Work out the finished part from the listing and answer in its coordinate system (mm). Coordinates: 2 decimals unless noted, no trailing zeros. Order: outer loops, then holes, each group sorted by start corner. A loop starts at its lowest first (then second) coordinate and runs counter-clockwise, first axis right, second up. Notation, with made-up numbers: (-14.75, 28.5) -> (-1.75, 28.5) arc R12 ccw to (-1.75, 33.5) -> close; hole circle Ø6 at (10, -36). An arc over 180 degrees is marked (long way). Answer as CSV lines item,"result". Start each with the question number.
Item 1: Straight lines are drawn through the part: L1, parallel to Z at x = -1.25, y = 1.2; L2, parallel to Y at x = 1, z = -8.25; L3, parallel to Y at x = -0.5, z = -12. For each, find the intervals that lie inside material, in ascending order.
Item 2: Each of these flat-tipped pins is pushed along its axis until it touches: pin 1 Ø0.5 at (x, y) = (-1, 1) entering from -Z; pin 2 Ø1.2 at (y, z) = (3, -9) entering from +X; pin 3 Ø1.2 at (y, z) = (2.5, -11.5) entering from -X. Where does it stop, or does it pass through?
Item 3: Section C-C (y = 1.65) is taken. Write down the section's boundary in (x, z).
Item 4: For a pull along Y with two mould halves and no side action, classify faces 1 (the face through (0.03, 3.08, -8.45)), 2 (the face through (0.028, 3.345, -8.182)), 3 (the face through (0, 1, -0.3)), 4 (the face through (0, 1, 0)) as pulls with the +Y half, pulls with the -Y half, needs draft (parallel to the pull), parting line crosses it, or undercut.
Item 5: Section A-A (x = 1.75) is taken. Write down the section's boundary in (y, z), then the cut area to 3 significant figures.
Item 6: Section B-B (z = -0.15) is taken. Write down the section's boundary in (x, y).
Item 7: Section D-D (z = -2.5) is taken. Write down the section's boundary in (x, y), then the cut area to 3 significant figures.
```python
from build123d import *

# Parameters (mm, degrees)
BASE_FLANGE1_DEPTH     = 2
CUT_EXTRUDE1_START     = -2
CUT_EXTRUDE1_OUTLINE_W = 0.3
CUT_EXTRUDE1_OUTLINE_H = 0.067712434
CUT_EXTRUDE1_DEPTH     = 4
SKETCH8_R              = 0.2
BOSS_EXTRUDE1_DEPTH    = 3.15


# Read off the part's stored shape, not the designer's step: Cut-Extrude1
# Sheet-metal steps are written as plain solids
with BuildPart() as part:
    # Sketch1 → Base-Flange1 (new, symmetric)
    with BuildSketch(Plane(origin=(0, 0, 0), x_dir=(0, 0, -1), z_dir=(1, 0, 0))):
        with BuildLine():
            Line((0, 0), (0, 1.852075023))
            ThreePointArc((0, 1.852075023), (0.09819474, 2.114588994), (0.344567924, 2.24821551))
            Line((0.344567924, 2.24821551), (16.24175994, 4.472715125))
            Line((16.24175994, 4.472715125), (16.283333998, 4.17560976))
            Line((16.283333998, 4.17560976), (0.386141981, 1.951110145))
            ThreePointArc((0.386141981, 1.951110145), (0.324548685, 1.917703516), (0.3, 1.852075023))
            Line((0.3, 1.852075023), (0.3, 0))
            Line((0.3, 0), (0, 0))
        make_face()
    extrude(amount=BASE_FLANGE1_DEPTH, both=True)

    # Cut-Extrude1 outline → Cut-Extrude1 (cut)
    with BuildSketch(Plane(origin=(0, 0, 0), x_dir=(0, 0, -1), z_dir=(1, 0, 0)).offset(CUT_EXTRUDE1_START)):
        with Locations((0.15, 0.033856217)):
            Rectangle(CUT_EXTRUDE1_OUTLINE_W, CUT_EXTRUDE1_OUTLINE_H)
    extrude(amount=CUT_EXTRUDE1_DEPTH, mode=Mode.SUBTRACT)

    # Sketch8 → Boss-Extrude1 (add, symmetric)
    with BuildSketch(Plane(origin=(0, 0, 0), x_dir=(0, 0, -1), z_dir=(1, 0, 0))):
        with Locations((0.15, 0.2)):
            Circle(SKETCH8_R)
    extrude(amount=BOSS_EXTRUDE1_DEPTH, both=True)


solid = part.part
```
Checked values:
1,L1,"z = -0.3 to 0"
1,L2,"y = 3.05 to 3.35"
1,L3,"y = 3.58 to 3.88"
2,pin 1,"stops at z = -0.3"
2,pin 2,"stops at x = 2"
2,pin 3,"passes through"
3,outline,"(-2, -0.3) -> (2, -0.3) -> (2, 0) -> (-2, 0) -> close"
4,face 1,"pulls with the -Y half"
4,face 2,"pulls with the +Y half"
4,face 3,"undercut"
4,face 4,"needs draft"
5,outline,"(0.33, -0.3) -> (1.85, -0.3) arc R0.1 cw to (1.95, -0.39) -> (4.18, -16.28) -> (4.47, -16.24) -> (2.25, -0.34) arc R0.4 ccw to (1.85, 0) -> (0.33, 0) arc R0.2 ccw (long way) to start"
5,area,"5.49 mm^2"
6,outline,"(-3.15, 0) -> (3.15, 0) -> (3.15, 0.4) -> (2, 0.4) -> (2, 2.16) -> (-2, 2.16) -> (-2, 0.4) -> (-3.15, 0.4) -> close"
7,outline,"(-2, 2.25) -> (2, 2.25) -> (2, 2.55) -> (-2, 2.55) -> close"
7,area,"1.21 mm^2"
